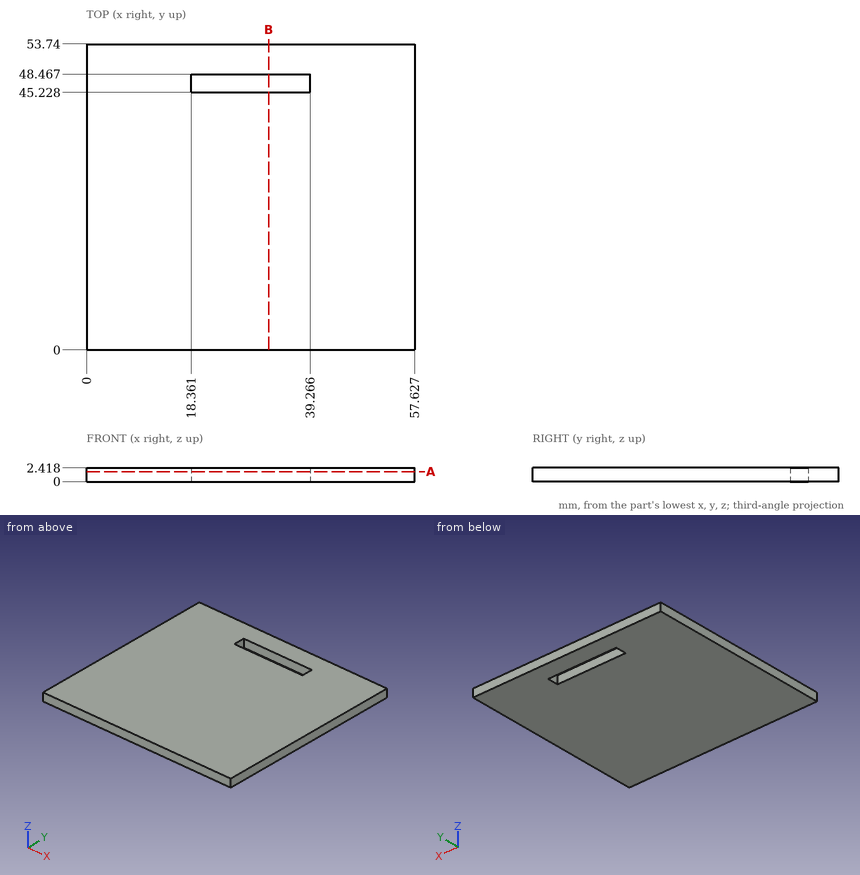
Study the drawing (mm; zero at the part's minimum x, y, z) and answer. Give positions to 0.01 mm unless a question says otherwise; leave off trailing zeros. Order: outer loops, then holes, each group sorted by start corner. A loop starts at its lowest first (then second) coordinate and runs counter-clockwise, first axis right, second up. Notation, with made-up numbers: (88, 37.25) - (119, 37.25) arc R8 ccw to (119, 49.25) - close; hole circle Ø10 at (-2.5, 3.25). An arc over 180 degrees is marked (long way). Use one line per item in the form item = value. Start each with the question number.
(1) A cutting plane is placed at A-A, the plane z = 1.75. Write down the section's boundary in (x, y).
(2) Consider line 1 (Y direction, x = 27, z = 0.2); line 2 (X direction, y = 46.5, z = 1). Determine where each line is inside the solid, lowest interval first. Write a range as from..to.
(3) A flat-ended cylindrical pin translates along its axis: pin 1 Ø0.7 at (x, z) = (32, 2) entering from -Y. Find the tip coordinate at first contact, or state that the pin passes through.
(4) A cutting plane is placed at B-B, the plane x = 32. Write down the section's boundary in (y, z).
Ans:
q1.outline = (0, 0) - (57.63, 0) - (57.63, 53.74) - (0, 53.74) - close; hole (18.36, 45.23) - (39.27, 45.23) - (39.27, 48.47) - (18.36, 48.47) - close
q2.line_1 = 0..45.23, 48.47..53.74
q2.line_2 = 0..18.36, 39.27..57.63
q3.pin_1 = 0
q4.outline = (0, 0) - (45.23, 0) - (45.23, 2.42) - (0, 2.42) - close; (48.47, 0) - (53.74, 0) - (53.74, 2.42) - (48.47, 2.42) - close
